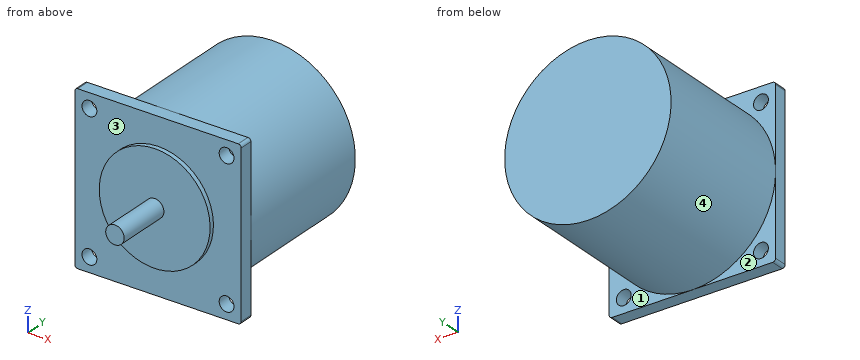
```python
from build123d import *

# Parameters (mm, degrees)
SKETCH_1_W                  = 57.2
SKETCH_1_H                  = 57.2
EXTRUDE_1_DEPTH             = 4.6
SKETCH_2_W                  = 28.6
SKETCH_2_H                  = 50
HOLE_WIZARD_5_1_5_1_1_D     = 5.1
HOLE_WIZARD_5_1_5_1_1_DEPTH = 54.6
FILLET_1_R                  = 1


with BuildPart() as part:
    # Эскиз1 → Бобышка-Вытянуть1 (new body)
    with BuildSketch(Plane.XZ.offset(4.6)):
        Rectangle(SKETCH_1_W, SKETCH_1_H)
    extrude(amount=-EXTRUDE_1_DEPTH)

    # Эскиз2 → Повернуть1 (revolve)
    with BuildSketch(Plane.XY, mode=Mode.PRIVATE) as revolve_1_sk:
        with Locations((14.3, 25)):
            Rectangle(SKETCH_2_W, SKETCH_2_H)
    revolve(revolve_1_sk.sketch.rotate(Axis((0, 50, 0), (0, -1, 0)), 270), axis=Axis((0, 50, 0), (0, -1, 0)))

    # Эскиз3 → Повернуть2 (revolve)
    with BuildSketch(Plane(origin=(0, 0, 0), x_dir=(-1, 0, 0), z_dir=(0, 0, -1)), mode=Mode.PRIVATE) as revolve_2_sk:
        Polygon((-3.175, -25.2), (0, -25.2), (0, -4.6), (-19.05, -4.6), (-19.05, -6.2), (-3.175, -6.2), align=None)
    revolve(revolve_2_sk.sketch.rotate(Axis((0, -25.2, 0), (0, 1, 0)), 270), axis=Axis((0, -25.2, 0), (0, 1, 0)))

    # Диаметр отверстия Ø5.1 (5.1)1
    with Locations(Plane(origin=(0, -4.6, 0), x_dir=(-1, 0, 0), z_dir=(0, -1, 0))):
        with Locations((23.57, 23.57), (23.57, -23.57), (-23.57, -23.57), (-23.57, 23.57)):
            Hole(HOLE_WIZARD_5_1_5_1_1_D / 2, depth=HOLE_WIZARD_5_1_5_1_1_DEPTH)

    # Скругление1
    fillet_1_edges = [part.edges().sort_by_distance(p)[0] for p in [
        (28.6, -2.3, 28.6),
        (28.6, -2.3, -28.6),
        (-28.6, -2.3, -28.6),
        (-28.6, -2.3, 28.6),
    ]]
    fillet(fillet_1_edges, radius=FILLET_1_R)


solid = part.part
```
Design review of the part built by this model. Coordinates are the model's own, in mm. Face numbers are marked on the shaded views. A direction names the side the tool comes from. Give positions to 0.01 mm unless a question says otherwise; leave off trailing zeros. Write each loop counter-clockwise with the first axis right and the second up, starting at its lowest first coordinate (ties: lowest second). Pieces come first, ordered by that corner, then holes. Notation, with made-up numbers: (-2.5, 63.5) -> (53.5, 63.5) arc R23 cw to (53.5, 97.5) -> close; hole circle Ø9 at (29, 68.25). An arc over 180 degrees is marked (long way). Answer in a Markdown table with one row per item.
(1) Consider section C-C (z = -7). State the section outline as (x, y) points.
Results:
| item | result |
|---|---|
| outline | (-28.6, -4.6) -> (-17.72, -4.6) -> (-17.72, -6.2) -> (17.72, -6.2) -> (17.72, -4.6) -> (28.6, -4.6) -> (28.6, 0) -> (27.73, 0) -> (27.73, 50) -> (-27.73, 50) -> (-27.73, 0) -> (-28.6, 0) -> close |
(2) Consider section D-D (y = 8.5). State the section outline as (x, z) points.
Results:
| item | result |
|---|---|
| outline | circle Ø57.2 at (0, 0) |
(3) Consider section B-B (x = 23.57). State the section outline as (y, z) points.
Results:
| item | result |
|---|---|
| outline | (-4.6, -28.6) -> (0, -28.6) -> (0, -26.12) -> (-4.6, -26.12) -> close; (-4.6, -21.02) -> (0, -21.02) -> (0, -16.2) -> (50, -16.2) -> (50, 16.2) -> (0, 16.2) -> (0, 21.02) -> (-4.6, 21.02) -> close; (-4.6, 26.12) -> (0, 26.12) -> (0, 28.6) -> (-4.6, 28.6) -> close |
(4) For the marked faces 1, 2, 3 and 4, list the 3-axis set-ups (+Z, -Z, +X, -X, +Y, -Y) from which the entire face can be reached by the end or side of a thin tool; tool diameter is ignored.
Results:
| item | result |
|---|---|
| face 1 | -Z, +X, +Y |
| face 2 | -Z, -X, +Y |
| face 3 | -Y |
| face 4 | +Y |
(5) Clearance check with flat-ended pins moving along their axes: pin 1 (12 mm diameter, centred on x = -20, y = 26.5, fed in from -Z); pin 2 (6.5 mm diameter, centred on x = -23.57, z = -23.57, fed in from -Y); pin 3 (12 mm diameter, centred on y = 28, z = -19.5, fed in from -X). State where each tip first meets the part, or that it passes through.
Results:
| item | result |
|---|---|
| pin 1 | z = -24.94 |
| pin 2 | y = -4.6 |
| pin 3 | x = -25.21 |
(6) To check wall thickness, follow probe 1 along Z at (x, y) = (-23.57, -2.4); probe 2 along X at (y, z) = (-1, 23). State the ranges of each line that lie inside material, in increasing order.
Results:
| item | result |
|---|---|
| probe 1 | -28.6 to -26.12, -21.02 to 21.02, 26.12 to 28.6 |
| probe 2 | -28.6 to -26.06, -21.08 to 21.08, 26.06 to 28.6 |
(7) Consider section A-A (z = -23.57). State the section outline as (x, y) points.
Results:
| item | result |
|---|---|
| outline | (-28.6, -4.6) -> (-26.12, -4.6) -> (-26.12, 0) -> (-28.6, 0) -> close; (-21.02, -4.6) -> (21.02, -4.6) -> (21.02, 0) -> (16.2, 0) -> (16.2, 50) -> (-16.2, 50) -> (-16.2, 0) -> (-21.02, 0) -> close; (26.12, -4.6) -> (28.6, -4.6) -> (28.6, 0) -> (26.12, 0) -> close |
